```python
from build123d import *

# Parameters (mm, degrees)
F0_W     = 508
F0_H     = 127.845764
F1_DEPTH = 12.7
F3_D     = 57.15
F5_D     = 30.48


with BuildPart() as f1:
    # F0 (on Front) → F1 (new body)
    with BuildSketch(Plane.XZ):
        Rectangle(F0_W, F0_H)
    extrude(amount=F1_DEPTH)

    # F3 (through all)
    with Locations(Plane.XZ.offset(12.7)):
        with Locations((-197.69825, 0), (198.532864, 0)):
            Hole(F3_D / 2)

    # F5 (through all)
    with Locations(Plane.XZ.offset(12.7)):
        with Locations((69.839768, 0)):
            Hole(F5_D / 2)


solid = f1.part
```
The model under review builds one solid part; all positions refer to its coordinate system, in mm. Coordinates: 2 decimals unless noted, no trailing zeros. Write each loop counter-clockwise with the first axis right and the second up, starting at its lowest first coordinate (ties: lowest second). Pieces come first, ordered by that corner, then holes. Notation, with made-up numbers: (79.5, -1) -> (89.5, -1) arc R12 cw to (89.5, 6) -> close; hole circle Ø1 at (8, 50.5). An arc over 180 degrees is marked (long way). One line per item, written item: value. Start each with the question number.
Q1. Add section B-B, the plane y = -7.5. Give the boundary of the cut face in (x, z) (3 decimals), then the cut area to 3 significant figures.
Q2. To check wall thickness, follow probe 1 along X at (y, z) = (-10.25, -26); probe 2 along X at (y, z) = (-9.5, 21); probe 3 along X at (y, z) = (-5.5, -9). State the ranges of each line that lie inside material, in increasing order.
Q3. Add section D-D, the plane x = 208.5. Give the boundary of the cut face in (y, z).
Q4. Add section A-A, the plane z = 0. Give the boundary of the cut face in (x, y).
Q5. The part is to be moulded in two halves that separate along X. For faces 1 (the face through (254, -6, -1)), 2 (the face through (-4, -12.7, 1)), 3 (the face through (55.304, -6.261, 4.578)), say which applies: +X half, -X half, draft (parallel to the pull), parting line (faces both ways), or undercut.
Q6. Add section C-C, the plane x = -205. Give the boundary of the cut face in (y, z), then the cut area to 3 significant figures.
Response:
1. outline: (-254, -63.923) -> (254, -63.923) -> (254, 63.923) -> (-254, 63.923) -> close; hole circle Ø57.15 at (-197.698, 0); hole circle Ø30.48 at (69.84, 0); hole circle Ø57.15 at (198.533, 0)
1. area: 59,100 mm²
2. probe 1: -254 to -209.55, -185.84 to 186.68, 210.39 to 254
2. probe 2: -254 to -217.08, -178.32 to 179.15, 217.91 to 254
2. probe 3: -254 to -224.82, -170.58 to 57.54, 82.14 to 171.41, 225.65 to 254
3. outline: (-12.7, -63.92) -> (0, -63.92) -> (0, -26.78) -> (-12.7, -26.78) -> close; (-12.7, 26.78) -> (0, 26.78) -> (0, 63.92) -> (-12.7, 63.92) -> close
4. outline: (-254, -12.7) -> (-226.27, -12.7) -> (-226.27, 0) -> (-254, 0) -> close; (-169.12, -12.7) -> (54.6, -12.7) -> (54.6, 0) -> (-169.12, 0) -> close; (85.08, -12.7) -> (169.96, -12.7) -> (169.96, 0) -> (85.08, 0) -> close; (227.11, -12.7) -> (254, -12.7) -> (254, 0) -> (227.11, 0) -> close
5. face 1: +X half
5. face 2: draft
5. face 3: undercut
6. outline: (-12.7, -63.92) -> (0, -63.92) -> (0, -27.63) -> (-12.7, -27.63) -> close; (-12.7, 27.63) -> (0, 27.63) -> (0, 63.92) -> (-12.7, 63.92) -> close
6. area: 922 mm²
